The model under review builds one solid part; all positions refer to its coordinate system, in mm. A direction names the side the tool comes from. Give positions to 0.01 mm unless a question says otherwise; leave off trailing zeros. Order: outer loops, then holes, each group sorted by start corner. A loop starts at its lowest first (then second) coordinate and runs counter-clockwise, first axis right, second up. Notation, with made-up numbers: (-10, 79) - (5, 79) arc R17 cw to (5, 91) - close; hole circle Ø9 at (69, 18.25). An arc over 180 degrees is marked (long way). Use CSV: the item, a comma, the result in double quotes. Start each with the question number.
1. Draft analysis for pull direction X (two halves, no side actions). For faces 1 (the flat face through (3, 40, 2)), 2 (the flat face through (31, 1, 3)), 3 (the flat face through (19, 45, 1)), state which applies: released by +X, released by -X, zero draft, split by the parting line, or undercut.
2. Take a section at C-C, the plane z = 3.1. State the section outline as (x, y) points.
3. Take a section at D-D, the plane x = 13.5. State the section outline as (y, z) points.
4. Take a section at B-B, the plane y = -37. State the section outline as (x, z) points, then the cut area to 3 significant figures.
5. For pin 1 (1 mm diameter, centred on x = 15.5, z = 3.5, fed in from -Y); pin 2 (1 mm diameter, centred on x = 13, z = 3, fed in from +Y); pin 3 (2 mm diameter, centred on x = 2, z = 2, fed in from +Y), all flat-tipped, find the tip position at first contact; note any pin that passes through.
6. Machinability: for faces 4 (the flat face through (-31, -1, 3)), 5 (the flat face through (18, 43.5, 3)), 6 (the flat face through (5, 42, 2)), which of the approach directions +Z, -Z, +X, -X, +Y, -Y give a long, thin tool a straight path to every point of the face, cutting with its end or side? Answer none if there is none.
7. Take a section at A-A, the plane x = -14. State the section outline as (y, z) points.
8. To check wall thickness, follow line 1 (Y direction, x = -14, z = 0.85); line 2 (Y direction, x = -14, z = 3); line 3 (Y direction, x = 13.5, z = 1). State the ranges of each line that lie inside material, in increasing order. Write a range as [from, to].
Autodesk Inventor part; units mm, degrees
ref_plane "YZ Plane" through (0, 0, 0) normal (1, 0, 0) x (0, 1, 0)
ref_plane "XZ Plane" through (0, 0, 0) normal (0, 1, 0) x (-1, 0, 0)
ref_plane "XY Plane" through (0, 0, 0) normal (0, 0, 1) x (1, 0, 0)
sketch "스케치1" plane through (0, 0, 0) normal (0, 0, 1) x (1, 0, 0)
  line L0 (-32.5, 45) -> (32.5, 45)
  line L1 (32.5, 45) -> (32.5, -45)
  line L2 (32.5, -45) -> (-32.5, -45)
  line L3 (-32.5, -45) -> (-32.5, 45)
  line L4 (-32.5, 45) -> (32.5, -45) construction
  line L5 (32.5, 45) -> (-32.5, -45) construction
  point P0 (0, 0)
  dimension "d0" = 65
  dimension "d1" = 90
extrude "돌출1" add sketch "스케치1" along normal blind 2
sketch "스케치3" plane through (0, 0, 2) normal (0, 0, 1) x (1, 0, 0)
  line L0 (-31, 43.5) -> (31, 43.5)
  line L1 (31, 43.5) -> (31, -43.5)
  line L2 (31, -43.5) -> (-31, -43.5)
  line L3 (-31, -43.5) -> (-31, 43.5)
  line L4 (-31, 43.5) -> (31, -43.5) construction
  line L5 (31, 43.5) -> (-31, -43.5) construction
  point P0 (0, 0)
  dimension "d8" = 62
  dimension "d9" = 87
extrude "돌출3" add sketch "스케치3" along normal blind 2
sketch "스케치5" plane through (0, 0, 4) normal (0, 0, 1) x (1, 0, 0)
  line L0 (32.5, 45) -> (-32.5, 45)
  line L1 (0, 45) -> (5, 45)
  line L2 (5, 45) -> (5, 40)
  line L3 (5, 40) -> (0, 40)
  line L4 (0, 40) -> (0, 45)
  point P0 (0, 0)
  dimension "d14" = 5
  dimension "d15" = 5
extrude "돌출4" cut sketch "스케치5" against normal blind 4
sketch "스케치6" plane through (0, 0, 4) normal (0, 0, 1) x (1, 0, 0)
  circle A0 centre (-14, 37) radius 2.5
  circle A1 centre (-14, -37) radius 2.5
  circle A2 centre (13.5, -19.5) radius 2.5
  point P0 (0, 0)
  dimension "d18" = 5
  dimension "d19" = 37
  dimension "d20" = 14
  dimension "d21" = 5
  dimension "d22" = 37
  dimension "d23" = 14
  dimension "d24" = 5
  dimension "d25" = 13.5
  dimension "d26" = 17.5
extrude "돌출5" cut sketch "스케치6" against normal blind 4
properties part number "upper"
Determined:
1,face 1,"undercut"
1,face 2,"released by +X"
1,face 3,"zero draft"
2,outline,"(-31, -43.5) - (31, -43.5) - (31, 43.5) - (5, 43.5) - (5, 40) - (0, 40) - (0, 43.5) - (-31, 43.5) - close; hole circle Ø5 at (-14, -37); hole circle Ø5 at (-14, 37); hole circle Ø5 at (13.5, -19.5)"
3,outline,"(-45, 0) - (-22, 0) - (-22, 4) - (-43.5, 4) - (-43.5, 2) - (-45, 2) - close; (-17, 0) - (45, 0) - (45, 2) - (43.5, 2) - (43.5, 4) - (-17, 4) - close"
4,outline,"(-32.5, 0) - (-16.5, 0) - (-16.5, 4) - (-31, 4) - (-31, 2) - (-32.5, 2) - close; (-11.5, 0) - (32.5, 0) - (32.5, 2) - (31, 2) - (31, 4) - (-11.5, 4) - close"
4,area,"234 mm²"
5,pin 1,"stops at y = -43.5"
5,pin 2,"stops at y = 43.5"
5,pin 3,"stops at y = 40"
6,face 4,"+Z, -X, +Y, -Y"
6,face 5,"+Z, +X, -X, +Y"
6,face 6,"+Z, -Z, +Y"
7,outline,"(-45, 0) - (-39.5, 0) - (-39.5, 4) - (-43.5, 4) - (-43.5, 2) - (-45, 2) - close; (-34.5, 0) - (34.5, 0) - (34.5, 4) - (-34.5, 4) - close; (39.5, 0) - (45, 0) - (45, 2) - (43.5, 2) - (43.5, 4) - (39.5, 4) - close"
8,line 1,"y = [-45, -39.5], [-34.5, 34.5], [39.5, 45]"
8,line 2,"y = [-43.5, -39.5], [-34.5, 34.5], [39.5, 43.5]"
8,line 3,"y = [-45, -22], [-17, 45]"
